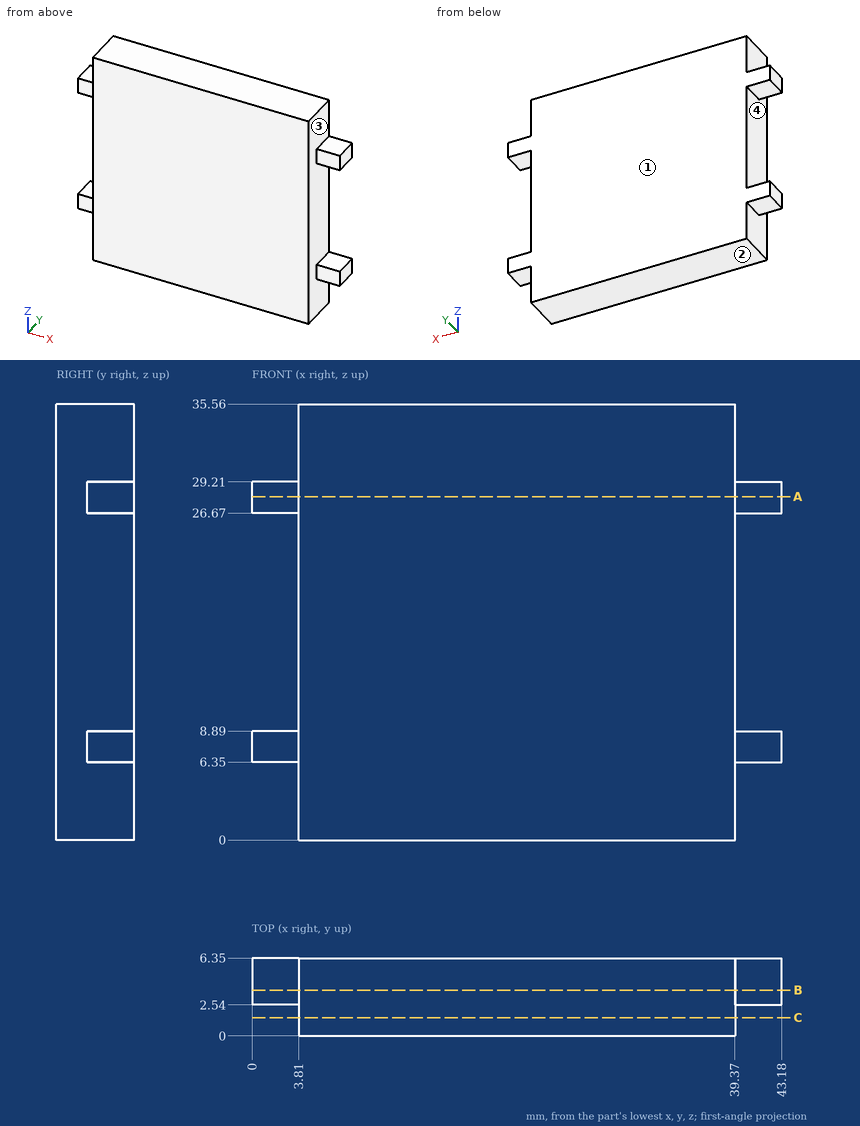
Check sheet for the drawn part. Datum: minimum x, y, z corner. Units: mm. Round coordinates to 2 decimals unless told otherwise and drop trailing zeros. Order: outer loops, then holes, each group sorted by start corner. A loop starts at its lowest first (then second) coordinate and runs counter-clockwise, first axis right, second up. Notation, with made-up numbers: (48.5, -33.75) -> (103.5, -33.75) arc R14 ccw to (103.5, -18.75) -> close; hole circle Ø5 at (83, -18.75). An arc over 180 degrees is marked (long way). Put each result on its own line as item: value.
1) Section check B-B (y = 3.75). Record the cut outline in (x, z), then the cut area to 3 significant figures.
Final values:
outline: (0, 6.35) -> (3.81, 6.35) -> (3.81, 0) -> (39.37, 0) -> (39.37, 6.35) -> (43.18, 6.35) -> (43.18, 8.89) -> (39.37, 8.89) -> (39.37, 26.67) -> (43.18, 26.67) -> (43.18, 29.21) -> (39.37, 29.21) -> (39.37, 35.56) -> (3.81, 35.56) -> (3.81, 29.21) -> (0, 29.21) -> (0, 26.67) -> (3.81, 26.67) -> (3.81, 8.89) -> (0, 8.89) -> close
area: 1,300 mm^2
2) Mould release check, pull along Z, two halves, no side actions. Record for the marked faces 1, 2, 3 and 4: +Z half, -Z half, draft (parallel to the pull), parting line (faces both ways), or undercut.
Final values:
face 1: draft
face 2: -Z half
face 3: undercut
face 4: undercut
3) Section check A-A (z = 28). Record the cut outline in (x, y).
Final values:
outline: (0, 2.54) -> (3.81, 2.54) -> (3.81, 0) -> (39.37, 0) -> (39.37, 2.54) -> (43.18, 2.54) -> (43.18, 6.35) -> (0, 6.35) -> close
4) Section check C-C (y = 1.5). Record the cut outline in (x, z), then the cut area to 3 significant figures.
Final values:
outline: (3.81, 0) -> (39.37, 0) -> (39.37, 35.56) -> (3.81, 35.56) -> close
area: 1,260 mm^2
5) Depth check by flat-ended pin: pin 1 (2 mm diameter, centred on y = 1, z = 28.5, fed in from +X); pin 2 (0.8 mm diameter, centred on x = 2, z = 28.5, fed in from -Y); pin 3 (3 mm diameter, centred on x = 41, y = 4, fed in from -Z). Enter the tip coordinate at first touch or a pass-through.
Final values:
pin 1: stops at x = 39.37
pin 2: stops at y = 2.54
pin 3: stops at z = 6.35
6) Material ranges on line 1 (Z direction, x = 2.5, y = 3.25); line 2 (X direction, y = 2.5, z = 16.5), recorded low to high.
Final values:
line 1: z = 6.35 to 8.89, 26.67 to 29.21
line 2: x = 3.81 to 39.37
